Geometry check sheet. Reference: the model listing, model coordinates, mm. A direction names the side the tool comes from. Coordinates: 2 decimals unless noted, no trailing zeros. Write each loop counter-clockwise with the first axis right and the second up, starting at its lowest first coordinate (ties: lowest second). Pieces come first, ordered by that corner, then holes. Notation, with made-up numbers: (-36.5, 52.25) -> (0.5, 52.25) arc R20 cw to (0.5, 80.25) -> close; hole circle Ø6 at (-36.5, 70.25). An arc over 180 degrees is marked (long way). Answer as CSV lines item,"result".
Autodesk Inventor part; units mm, degrees
ref_plane "YZ Plane" through (0, 0, 0) normal (1, 0, 0) x (0, 1, 0)
ref_plane "XZ Plane" through (0, 0, 0) normal (0, 1, 0) x (-1, 0, 0)
ref_plane "XY Plane" through (0, 0, 0) normal (0, 0, 1) x (1, 0, 0)
sketch "Sketch1" plane through (0, 0, 0) normal (0, 1, 0) x (-1, 0, 0)
  line L0 (-2, 0) -> (-35.8284, 0)
  line L1 (-37.8284, -2) -> (-37.8284, -18)
  line L2 (-10, -37) -> (-2, -37)
  line L3 (0, -35) -> (0, -2)
  line L4 (-37, -36.9907) -> (-37, -19.9907) construction
  line L5 (-35.8284, -20) -> (-27.8284, -20)
  line L6 (0, -37) -> (-10, -37) construction
  line L7 (-11.4142, -36.4142) -> (-27.8284, -20)
  arc A0 (-37.8284, -18) -> (-35.8284, -20) centre (-35.8284, -18) ccw
  arc A1 (-35.8284, 0) -> (-37.8284, -2) centre (-35.8284, -2) ccw
  arc A2 (-2, -37) -> (0, -35) centre (-2, -35) ccw
  arc A3 (0, -2) -> (-2, 0) centre (-2, -2) ccw
  arc A4 (-11.4142, -36.4142) -> (-10, -37) centre (-10, -35) ccw
  point P0 (0, 0)
  point P1 (-37.8284, 0)
  point P2 (-37.8284, -20)
  dimension "d0" = 37
  dimension "d2" = 17
  dimension "d3" = 10
  dimension "d4" = 10
  dimension "d5" = 2
  dimension "d6" = 2
extrude "Extrusion1" add sketch "Sketch1" along normal blind 1.65
sketch "Sketch2" plane through (0, 0, 0) normal (0, -1, 0) x (1, 0, 0)
  line L0 (27.8284, -20) -> (35.8284, -20)
  line L1 (37.8284, -18) -> (37.8284, -2)
  line L2 (37.8105, 0.5) -> (30.8284, 0.5)
  line L3 (30.8284, 0.5) -> (30.8284, -20)
  line L4 (37.8105, -20.5) -> (37.8105, 0.5)
  line L5 (41.55, -10) -> (26.7279, -10) construction
  line L6 (37.8105, -20.5) -> (30.8284, -20.5)
  line L7 (30.8284, -20.5) -> (30.8284, -20)
  point P0 (0, 0)
  point P1 (37.8284, -10)
  dimension "d11" = 10.5
extrude "Extrusion2" add sketch "Sketch2" along normal blind 8.3
sketch "Sketch3" plane through (0, 1.65, 0) normal (0, 1, 0) x (1, 0, 0)
  line L0 (0, 35) -> (0, 2)
  line L1 (2, 0) -> (35.8284, 0)
  line L2 (37.8284, 2) -> (37.8284, 18)
  line L3 (6, 38.3943) -> (6, -5.9246) construction
  line L4 (6, 0) -> (6, 1.25) construction
  circle A0 centre (6, 1.25) radius 0.37
  circle A1 centre (6, 3.85) radius 0.37
  circle A2 centre (6, 6.45) radius 0.37
  circle A3 centre (6, 9.05) radius 0.37
  circle A4 centre (6, 11.65) radius 0.37
  circle A5 centre (6, 14.25) radius 0.37
  circle A6 centre (6, 16.85) radius 0.37
  circle A7 centre (6, 19.45) radius 0.37
  circle A8 centre (6, 22.05) radius 0.37
  circle A9 centre (6, 24.65) radius 0.37
  circle A10 centre (6, 27.25) radius 0.37
  circle A11 centre (6, 29.85) radius 0.37
  circle A12 centre (6, 32.45) radius 0.37
  circle A13 centre (6, 35.05) radius 0.37
  line L5 (35.8284, 20) -> (27.8284, 20)
  line L6 (10, 37) -> (2, 37)
  line L7 (37.8284, 10) -> (29.2284, 10) construction
  line L8 (29.2284, 10) -> (29.2284, 28.7418) construction
  line L9 (29.2284, 20) -> (29.2284, 18.75) construction
  line L10 (29.2284, 0) -> (29.2284, 1.25) construction
  circle A14 centre (29.2284, 1.25) radius 0.37
  circle A15 centre (29.2284, 3.85) radius 0.37
  circle A16 centre (29.2284, 6.45) radius 0.37
  circle A17 centre (29.2284, 9.05) radius 0.37
  circle A18 centre (29.2284, 11.65) radius 0.37
  circle A19 centre (29.2284, 14.25) radius 0.37
  circle A20 centre (29.2284, 16.85) radius 0.37
  circle A21 centre (29.2284, 19.45) radius 0.37
  point P0 (0, 0)
  dimension "d16" = 1.25
  dimension "d17" = 0.74
  dimension "d20" = 2.6
  dimension "d27" = 8.6
  dimension "d37" = 0.74
  dimension "d40" = 2.6
  dimension "d50" = 6
extrude "Extrusion3" add sketch "Sketch3" along normal blind 5
sketch "Sketch4" plane through (0, 0, 0) normal (0, -1, 0) x (1, 0, 0)
  line L0 (30.8284, 0) -> (2, 0)
  line L1 (0, 0) -> (7, 0) construction
  line L2 (7, 0) -> (27, 0)
  line L3 (27, 0) -> (27, -20)
  line L4 (27, -20) -> (7, -20)
  line L5 (7, -20) -> (7, 0)
  dimension "d45" = 7
  dimension "d46" = 20
  dimension "d47" = 20
extrude "Extrusion4" add sketch "Sketch4" along normal blind 5.7
equation "\"d47\" = d46"
properties part number "Adaptador TB6612FNG"
Item 1: Set-up check for faces 5 (the flat face through (34.8, 0, 0.3)), 6 (the flat face through (17, -5.7, -10)), 7 (the flat face through (17, -3, -20)), 8 (the cylindrical face through (37.227, 0.813, -19.43)): record each of +Z, -Z, +X, -X, +Y, -Y from which the full face is reachable in a straight line by a thin tool's end or side.
Responses:
face 5,"+Z, +X, +Y"
face 6,"+Z, -Z, -X, -Y"
face 7,"-Z, -X, -Y"
face 8,"-Z, +X, +Y"
Item 2: Release check for a two-part mould opening along X. For faces 1 (the flat face through (30.828, -4, -10)), 2 (the flat face through (27, -3, -10)), 3 (the flat face through (37.828, 1, -10)), 4 (the flat face through (0, 1, -19)) record: +X half, -X half, draft (parallel to the pull), parting line (faces both ways), or undercut.
Responses:
face 1,"undercut"
face 2,"undercut"
face 3,"+X half"
face 4,"-X half"
Item 3: Cross-section at B-B, the plane y = 3.5. Count the separate pieces of the cut face and the enclosed holes in it, plus the area to 3 significant figures.
Responses:
separate pieces,"22"
enclosed holes,"0"
area,"9.46 mm2"
Item 4: Cross-section at C-C, the plane x = 33.5. Record the cut outline in (y, z), plus the area to 3 significant figures.
Responses:
outline,"(-8.3, -20.5) -> (0, -20.5) -> (0, -20) -> (1.65, -20) -> (1.65, 0) -> (0, 0) -> (0, 0.5) -> (-8.3, 0.5) -> close"
area,"207 mm2"
Item 5: Cross-section at A-A, the plane y = -5. Record the cut outline in (x, z), plus the area to 3 significant figures.
Responses:
outline,"(7, -20) -> (27, -20) -> (27, 0) -> (7, 0) -> close; (30.83, -20.5) -> (37.81, -20.5) -> (37.81, 0.5) -> (30.83, 0.5) -> close"
area,"547 mm2"
Item 6: Thickness scan on probe 1 along X at (y, z) = (-3.5, -8); probe 2 along Y at (x, z) = (32, -14.5); probe 3 along Y at (x, z) = (26.5, -11). Record the ranges inside material, lowest first.
Responses:
probe 1,"x = 7 to 27, 30.83 to 37.81"
probe 2,"y = -8.3 to 1.65"
probe 3,"y = -5.7 to 1.65"
Item 7: Cross-section at D-D, the plane z = -31. Record the cut outline in (x, y), plus the area to 3 significant figures.
Responses:
outline,"(0, 0) -> (16.83, 0) -> (16.83, 1.65) -> (0, 1.65) -> close"
area,"27.8 mm2"
Item 8: Depth check by flat-ended pin: pin 1 Ø4 at (y, z) = (4.5, -15) entering from -X; pin 2 Ø5 at (x, z) = (8, -18) entering from +Y; pin 3 Ø15.5 at (x, z) = (11.5, -13) entering from -Y; pin 4 Ø4 at (y, z) = (-4.5, -9.5) entering from -X. Enter the tip coordinate at first touch or a pass-through.
Responses:
pin 1,"stops at x = 5.63"
pin 2,"stops at y = 6.65"
pin 3,"stops at y = -5.7"
pin 4,"stops at x = 7"
